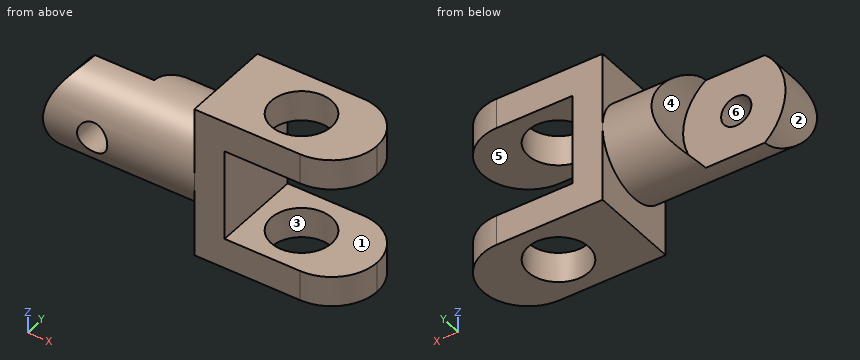
```python
from build123d import *

# Parameters (mm, degrees)
BOSS_EXTRUDE1_DEPTH      = 4.70535
BOSS_EXTRUDE1_DEPTH_BACK = 4.70535
SKETCH2_R                = 4.70535
BOSS_EXTRUDE2_DEPTH      = 17.25168
CUT_EXTRUDE3_DEPTH       = 10.4107
SKETCH5_R                = 5.900934737
CUT_EXTRUDE4_DEPTH       = 4.70408
SKETCH6_R                = 1.56718
CUT_EXTRUDE5_DEPTH       = 5.706620123
FILLET1_R                = 4.70408
SKETCH7_R                = 3.1369
CUT_EXTRUDE6_DEPTH       = 16.68196


with BuildPart() as part:
    # Sketch1 → Boss-Extrude1 (new body, two sides)
    with BuildSketch(Plane(origin=(0, 0, 0), x_dir=(1, 0, 0), z_dir=(0, 1, 0))) as boss_extrude1_sk:
        Polygon((-12.54506, 4.70408), (0, 4.70408), (0, 7.84098), (-15.68196, 7.84098), (-15.68196, -7.84098), (0, -7.84098), (0, -4.70408), (-12.54506, -4.70408), align=None)
    extrude(amount=BOSS_EXTRUDE1_DEPTH)
    extrude(boss_extrude1_sk.sketch, amount=-BOSS_EXTRUDE1_DEPTH_BACK)

    # Sketch2 → Boss-Extrude2 (add)
    with BuildSketch(Plane.ZY.offset(15.68196)):
        Circle(SKETCH2_R)
    extrude(amount=BOSS_EXTRUDE2_DEPTH)

    # Sketch3 → Cut-Extrude3 (cut, through all)
    with BuildSketch(Plane(origin=(0, 4.70535, 0), x_dir=(1, 0, 0), z_dir=(0, 1, 0))):
        with BuildLine():
            Line((-25.09266, 6.2738), (-33.67290655, 6.2738))
            Line((-33.67290655, 6.2738), (-33.67290655, -6.2738))
            Line((-33.67290655, -6.2738), (-25.09266, -6.2738))
            ThreePointArc((-25.09266, -6.2738), (-31.36646, 0), (-25.09266, 6.2738))
        make_face()
    extrude(amount=-CUT_EXTRUDE3_DEPTH, mode=Mode.SUBTRACT)

    # Sketch5 → Cut-Extrude4 (cut)
    with BuildSketch(Plane(origin=(0, 4.70535, 0), x_dir=(1, 0, 0), z_dir=(0, 1, 0))):
        with Locations((-26.65984, 0)):
            Circle(SKETCH5_R)
    extrude(amount=-CUT_EXTRUDE4_DEPTH, mode=Mode.SUBTRACT)

    # Sketch6 → Cut-Extrude5 (cut, through all)
    with BuildSketch(Plane(origin=(0, 0.00127, 0), x_dir=(1, 0, 0), z_dir=(0, 1, 0))):
        with Locations((-26.26868, 0)):
            Circle(SKETCH6_R)
    extrude(amount=-CUT_EXTRUDE5_DEPTH, mode=Mode.SUBTRACT)

    # Fillet1
    fillet1_edges = [part.edges().sort_by_distance(p)[0] for p in [
        (0, -4.70535, -6.27253),
        (0, -4.70535, 6.27253),
        (0, 4.70535, -6.27253),
        (0, 4.70535, 6.27253),
    ]]
    fillet(fillet1_edges, radius=FILLET1_R)

    # Sketch7 → Cut-Extrude6 (cut, through all)
    with BuildSketch(Plane.XY.offset(7.84098)):
        with Locations((-7.84098, 0)):
            Circle(SKETCH7_R)
    extrude(amount=-CUT_EXTRUDE6_DEPTH, mode=Mode.SUBTRACT)


solid = part.part
```
Read the model definition and answer for the solid it produces. Units are mm, in the model's axes. Face numbers are marked on the shaded views. A direction names the side the tool comes from. Give positions to 0.01 mm unless a question says otherwise; leave off trailing zeros. Write each loop counter-clockwise with the first axis right and the second up, starting at its lowest first coordinate (ties: lowest second). Pieces come first, ordered by that corner, then holes. Notation, with made-up numbers: (61.25, -6.5) -> (98.25, -6.5) arc R18 ccw to (98.25, 22.5) -> close; hole circle Ø9 at (78.5, -9.5). An arc over 180 degrees is marked (long way). Answer as a JSON object with one key per item and string values.
1) A tool of negligible diameter and unlimited length cuts with its end or side. For the marked faces 4, 5 and 6, from which of +Z, -Z, +X, -X, +Y, -Y can it reach the whole face along a straight path? Write none if from no direction.
Findings below:
{"face 4": "-X, +Y", "face 5": "+X, +Y, -Y", "face 6": "+Y, -Y"}
2) Straight lines are drawn through the part: probe 1 along Z at (x, y) = (-4, -3.75); probe 2 along X at (y, z) = (-3.6, 0); probe 3 along Z at (x, y) = (-18, 3.5). For each, find the intervals that lie inside material, in ascending order. Write a range as from..to.
Findings below:
{"probe 1": "z = -7.84..-4.7, 4.7..7.84", "probe 2": "x = -31.37..-27.84, -24.7..-12.55", "probe 3": "z = -3.14..3.14"}
3) Flat-ended cylindrical pins translate along their axes: pin 1 Ø1 at (x, z) = (-22, 6) entering from +Y; pin 2 Ø6 at (x, z) = (-25, 6) entering from -Y; pin 3 Ø4 at (x, z) = (-26.5, -3.5) entering from -Y; pin 4 Ø3 at (y, z) = (-2, 1) entering from +X. Find the tip coordinate at first contact, or state that the pin passes through.
Findings below:
{"pin 1": "passes through", "pin 2": "stops at y = -3.62", "pin 3": "stops at y = -4.46", "pin 4": "stops at x = -12.55"}
4) Section D-D on y = 1.5 is taken. Write down the section's boundary in (x, z), then the cut area to 3 significant figures.
Findings below:
{"outline": "(-22.8, -4.46) -> (-15.68, -4.46) -> (-15.68, -7.84) -> (-10.6, -7.84) -> (-10.6, -4.7) -> (-12.55, -4.7) -> (-12.55, 4.7) -> (-10.6, 4.7) -> (-10.6, 7.84) -> (-15.68, 7.84) -> (-15.68, 4.46) -> (-22.8, 4.46) arc R5.9 cw to start; (-5.09, -7.84) -> (-0.25, -7.84) -> (-0.25, -4.7) -> (-5.09, -4.7) -> close; (-5.09, 4.7) -> (-0.25, 4.7) -> (-0.25, 7.84) -> (-5.09, 7.84) -> close", "area": "143 mm^2"}
5) For a pull along Z with two mould halves and no side action, classify the marked faces 1, 2 and 3 as pulls with the +Z half, pulls with the -Z half, needs draft (parallel to the pull), parting line crosses it, or undercut.
Findings below:
{"face 1": "undercut", "face 2": "parting line crosses it", "face 3": "needs draft"}
6) Section B-B on y = -0.75 is taken. Write down the section's boundary in (x, z), then the cut area to 3 significant figures.
Findings below:
{"outline": "(-29.31, -4.65) -> (-15.68, -4.65) -> (-15.68, -7.84) -> (-10.89, -7.84) -> (-10.89, -4.7) -> (-12.55, -4.7) -> (-12.55, 4.7) -> (-10.89, 4.7) -> (-10.89, 7.84) -> (-15.68, 7.84) -> (-15.68, 4.65) -> (-29.31, 4.65) arc R6.27 ccw to start; (-4.8, -7.84) -> (-0.06, -7.84) -> (-0.06, -4.7) -> (-4.8, -4.7) -> close; (-4.8, 4.7) -> (-0.06, 4.7) -> (-0.06, 7.84) -> (-4.8, 7.84) -> close; hole circle Ø3.13 at (-26.27, 0)", "area": "221 mm^2"}
7) Section A-A on x = -12 is taken. Write down the section's boundary in (y, z).
Findings below:
{"outline": "(-4.71, -7.84) -> (4.71, -7.84) -> (4.71, -4.7) -> (-4.71, -4.7) -> close; (-4.71, 4.7) -> (4.71, 4.7) -> (4.71, 7.84) -> (-4.71, 7.84) -> close"}
8) Section C-C on z = 1 is taken. Write down the section's boundary in (x, y), then the cut area to 3 significant figures.
Findings below:
{"outline": "(-31.29, -4.6) -> (-27.48, -4.6) -> (-27.48, 0) -> (-31.29, 0) -> close; (-25.06, -4.6) -> (-15.68, -4.6) -> (-15.68, -4.71) -> (-12.55, -4.71) -> (-12.55, 4.71) -> (-15.68, 4.71) -> (-15.68, 4.6) -> (-20.84, 4.6) -> (-20.84, 0) -> (-25.06, 0) -> close", "area": "114 mm^2"}
